```python
from build123d import *

# Parameters (mm, degrees)
SKETCH1_W               = 14
SKETCH1_H               = 14
BOSS_EXTRUDE1_DEPTH     = 10
SKETCH2_R               = 43.1
CUT_EXTRUDE1_DEPTH      = 8
CUT_EXTRUDE1_DEPTH_BACK = 8
SKETCH3_W               = 9.8
SKETCH3_H               = 9.8
BOSS_EXTRUDE2_DEPTH     = 15
SKETCH5_R               = 36
CUT_EXTRUDE2_DEPTH      = 8
CUT_EXTRUDE2_DEPTH_BACK = 8


with BuildPart() as part:
    # Sketch1 → Boss-Extrude1 (new body)
    with BuildSketch(Plane(origin=(0, 0, 0), x_dir=(1, 0, 0), z_dir=(0, 1, 0))):
        Rectangle(SKETCH1_W, SKETCH1_H)
    extrude(amount=BOSS_EXTRUDE1_DEPTH)

    # Sketch2 → Cut-Extrude1 (cut, two sides)
    with BuildSketch(Plane.XY) as cut_extrude1_sk:
        with Locations((0, -37)):
            Circle(SKETCH2_R)
    extrude(amount=CUT_EXTRUDE1_DEPTH, mode=Mode.SUBTRACT)
    extrude(cut_extrude1_sk.sketch, amount=-CUT_EXTRUDE1_DEPTH_BACK, mode=Mode.SUBTRACT)

    # Sketch3 → Boss-Extrude2 (add)
    with BuildSketch(Plane(origin=(0, 10, 0), x_dir=(1, 0, 0), z_dir=(0, 1, 0))):
        Rectangle(SKETCH3_W, SKETCH3_H)
    extrude(amount=-BOSS_EXTRUDE2_DEPTH)

    # Sketch5 → Cut-Extrude2 (cut, two sides)
    with BuildSketch(Plane.XY) as cut_extrude2_sk:
        with Locations((0, -37)):
            Circle(SKETCH5_R)
    extrude(amount=CUT_EXTRUDE2_DEPTH, mode=Mode.SUBTRACT)
    extrude(cut_extrude2_sk.sketch, amount=-CUT_EXTRUDE2_DEPTH_BACK, mode=Mode.SUBTRACT)


solid = part.part
```
Read the model definition and answer for the solid it produces. Units are mm, in the model's axes. Round coordinates to 2 decimals unless told otherwise and drop trailing zeros. Write each loop counter-clockwise with the first axis right and the second up, starting at its lowest first coordinate (ties: lowest second). Pieces come first, ordered by that corner, then holes. Notation, with made-up numbers: (-19.75, 78.25) - (14.25, 78.25) arc R21 cw to (14.25, 93.25) - close; hole circle Ø8 at (-20.5, 48.5). An arc over 180 degrees is marked (long way). One line per item, written item: value.
Q1. Find section C-C (y = 2.25). Determine the outline of the cut face in (x, z).
The answers:
outline: (-4.9, -4.9) - (4.9, -4.9) - (4.9, 4.9) - (-4.9, 4.9) - close
Q2. Find section D-D (z = -5.75). Determine the outline of the cut face in (x, y).
The answers:
outline: (-7, 5.53) arc R43.1 cw to (7, 5.53) - (7, 10) - (-7, 10) - close
Q3. Each of these flat-tipped pins is pushed along its axis until it touches: P1, Ø2, axis at y = 3.5, z = 0.5, coming from the -X side; P2, Ø6, axis at x = 0.5, y = 0.5, coming from the +Z side. Where does it stop, or does it pass through?
The answers:
P1: stops at x = -4.9
P2: stops at z = 4.9
Q4. For a pull along X with two mould halves and no side action, classify faces 1 (the cylindrical face through (0, -1, 0)), 2 (the flat face through (7, 8, 0)), 3 (the flat face through (0, 8, -7)), 4 (the flat face through (-7, 8, 0)) as pulls with the +X half, pulls with the -X half, needs draft (parallel to the pull), parting line crosses it, or undercut.
The answers:
face 1: undercut
face 2: pulls with the +X half
face 3: needs draft
face 4: pulls with the -X half
Q5. Find section A-A (z = -3). Determine the outline of the cut face in (x, y), and give its area (3 significant figures).
The answers:
outline: (-7, 5.53) arc R43.1 cw to (-4.9, 5.82) - (-4.9, -1.34) arc R36 cw to (4.9, -1.34) - (4.9, 5.82) arc R43.1 cw to (7, 5.53) - (7, 10) - (-7, 10) - close
area: 127 mm2
Q6. Straight lines are drawn through the part: line 1 (X direction, y = 3, z = 4.5); line 2 (Y direction, x = 0.5, z = 1.25). For each, find the intervals that lie inside material, in ascending order. Write a range as from..to.
The answers:
line 1: x = -4.9..4.9
line 2: y = -1..10
Q7. Find section B-B (x = -2.25). Determine the outline of the cut face in (y, z).
The answers:
outline: (-1.07, -4.9) - (6.04, -4.9) - (6.04, -7) - (10, -7) - (10, 7) - (6.04, 7) - (6.04, 4.9) - (-1.07, 4.9) - close
